Geometry check sheet. Reference: the model listing, model coordinates, mm. A direction names the side the tool comes from. Round coordinates to 2 decimals unless told otherwise and drop trailing zeros. Write each loop counter-clockwise with the first axis right and the second up, starting at its lowest first coordinate (ties: lowest second). Pieces come first, ordered by that corner, then holes. Notation, with made-up numbers: (54, 52.5) - (78, 52.5) arc R4 cw to (78, 58.5) - close; hole circle Ø4 at (16, 89). An arc over 180 degrees is marked (long way). Return JSON: item names as keys, results as strings. Group by question number.
Autodesk Inventor part; units mm, degrees
ref_plane "YZ Plane" through (0, 0, 0) normal (1, 0, 0) x (0, 1, 0)
ref_plane "XZ Plane" through (0, 0, 0) normal (0, 1, 0) x (-1, 0, 0)
ref_plane "XY Plane" through (0, 0, 0) normal (0, 0, 1) x (1, 0, 0)
sketch "Sketch1" plane through (0, 0, 0) normal (0, 0, 1) x (1, 0, 0)
  line L0 (0, 0) -> (-30, 0) construction
  line L1 (0, 10) -> (-30, 10)
  line L2 (-30, -10) -> (0, -10)
  arc A0 (0, -10) -> (0, 10) centre (0, 0) ccw
  arc A1 (-30, 10) -> (-30, -10) centre (-30, 0) ccw
  circle A2 centre (-30, 0) radius 1.55
  circle A3 centre (0, 0) radius 1.55
  line L3 (-30, 10) -> (0, 10)
  line L4 (0, 10) -> (0, 15)
  line L5 (0, 15) -> (-30, 15)
  line L6 (-30, 15) -> (-30, 10)
  point P0 (-15, 0)
  dimension "d0" = 20
  dimension "d1" = 30
  dimension "d2" = 3.1
  dimension "d3" = 3.1
  dimension "d7" = 5
extrude "Extrusion1" add sketch "Sketch1" along normal blind 20
sketch "Sketch3" plane through (0, 0, 0) normal (1, 0, 0) x (0, 1, 0)
  circle A0 centre (8, 10) radius 1
  point P0 (0, 0)
  dimension "d8" = 2
  dimension "d9" = 8
  dimension "d10" = 10
extrude "Extrusion2" cut sketch "Sketch3" along normal mid plane 100
1. Section check D-D (y = -3.5). Enter the section's corners in (x, z), and give its area (3 significant figures).
2. Section check A-A (z = 8.5). Enter the section's corners in (x, y), and give its area (3 significant figures).
3. Material ranges on line 1 along Z through (x, y) = (-7, 8); line 2 along Y through (x, z) = (-7, 10); line 3 along Z through (x, y) = (1.5, 7.5), recorded low to high.
4. Mould release check, pull along X, two halves, no side actions. Record for faces 4 (the face through (-15, 3, 20)), 5 (the face through (0.715, 1.375, 9.86)), 6 (the face through (10, 0, 10)): pulls with the +X half, pulls with the -X half, needs draft (parallel to the pull), parting line crosses it, or undercut.
5. Depth check by flat-ended pin: pin 1 Ø5.5 at (y, z) = (12, 11) entering from -X; pin 2 Ø2 at (x, y) = (-4, 9.5) entering from -Z; pin 3 Ø5 at (y, z) = (7.5, 5.5) entering from +X; pin 4 Ø8 at (y, z) = (10.5, 3) entering from -X. Enter the tip coordinate at first touch or a pass-through.
6. Tool access check on faces 1 (the face through (-30, 13, 10)), 2 (the face through (-15, 3, 0)), 3 (the face through (0, 12, 10)). Record the directions out of +Z, -Z, +X, -X, +Y, -Y that give a thin tool (end or side, any length) a straight path to the whole face; none if there is none.
7. Section check B-B (y = 0.75). Enter the section's corners in (x, z), and give its area (3 significant figures).
8. Section check C-C (y = 8). Enter the section's corners in (x, z), and give its area (3 significant figures).
Result sheet:
{
 "1": {"outline": "(-39.37, 0) - (9.37, 0) - (9.37, 20) - (-39.37, 20) - close", "area": "975 mm²"},
 "2": {"outline": "(-30, -10) - (0, -10) arc R10 ccw to (0, 10) - (0, 15) - (-30, 15) - (-30, 10) arc R10 ccw to start; hole circle Ø3.1 at (-30, 0); hole circle Ø3.1 at (0, 0)", "area": "1,050 mm²"},
 "3": {"line 1": "z = 0 to 9, 11 to 20", "line 2": "y = -10 to 7, 9 to 15", "line 3": "z = 0 to 9.13, 10.87 to 20"},
 "4": {"face 4": "needs draft", "face 5": "undercut", "face 6": "pulls with the +X half"},
 "5": {"pin 1": "stops at x = -33.8", "pin 2": "stops at z = 0", "pin 3": "stops at x = 8.66", "pin 4": "stops at x = -37.6"},
 "6": {"face 1": "+Z, -Z, -X, +Y", "face 2": "-Z, +X, -X, +Y, -Y", "face 3": "+Z, -Z, +X, +Y"},
 "7": {"outline": "(-39.97, 0) - (-31.36, 0) - (-31.36, 20) - (-39.97, 20) - close; (-28.64, 0) - (-1.36, 0) - (-1.36, 20) - (-28.64, 20) - close; (1.36, 0) - (9.97, 0) - (9.97, 20) - (1.36, 20) - close", "area": "890 mm²"},
 "8": {"outline": "(-36, 0) - (6, 0) - (6, 9) - (-36, 9) - close; (-36, 11) - (6, 11) - (6, 20) - (-36, 20) - close", "area": "756 mm²"}
}
